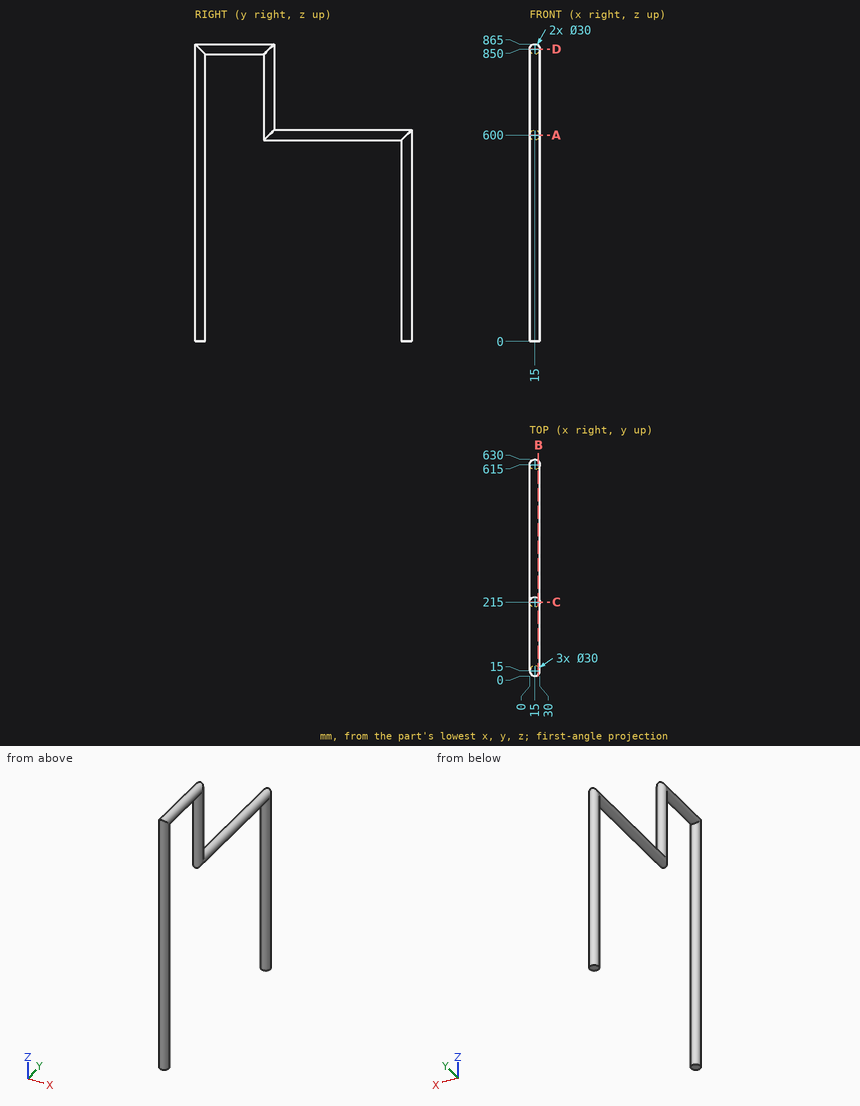
Could you check a few things on this drawing? It's one solid part, dimensions in mm from its lowest x, y, z. Coordinates: 2 decimals unless noted, no trailing zeros. Write each loop counter-clockwise with the first axis right and the second up, starting at its lowest first coordinate (ties: lowest second). Pieces come first, ordered by that corner, then holes. Notation, with made-up numbers: (-1.75, 49.5) - (28.25, 49.5) arc R23 cw to (28.25, 70.5) - close; hole circle Ø6 at (77, 20). An arc over 180 degrees is marked (long way). Return JSON: item names as keys, results as strings. Group by question number.
Item 1: If we section it at D-D (z = 850): Write out the boundary of the cut face in (x, y).
Item 2: I'm going to push flat-ended pins straight in: pin 1 Ø10 at (x, y) = (20, 438.5) entering from +Z; pin 2 Ø10 at (x, z) = (14.5, 307.5) entering from +Y; pin 3 Ø1.5 at (x, z) = (12, 713) entering from -Y; pin 4 Ø6 at (x, z) = (21.5, 559) entering from -Y. Where does each tip first touch, or does it pass through?
Item 3: If we section it at A-A (z = 600): Write out the boundary of the cut face in (x, y), then the cut area to 3 significant figures.
Item 4: Please list where these lines run through material, in increasing order: probe 1 along Y at (x, z) = (13, 750.5); probe 2 along Y at (x, z) = (14, 261); probe 3 along Z at (x, y) = (13.5, 574).
Item 5: If we section it at B-B (x = 25.25): Write out the boundary of the cut face in (y, z).
Item 6: If we section it at C-C (y = 215): Write out the boundary of the cut face in (x, z), then the cut area to 3 significant figures.
Return value:
{
 "1": {"outline": "(0, 15) arc R15 ccw to (30, 15) - (30, 215) arc R15 ccw to (0, 215) - close"},
 "2": {"pin 1": "stops at z = 615", "pin 2": "stops at y = 630", "pin 3": "stops at y = 0.17", "pin 4": "stops at y = 0.41"},
 "3": {"outline": "circle Ø30 at (15, 15); (0, 215) arc R15 ccw to (30, 215) - (30, 615) arc R15 ccw to (0, 615) - close", "area": "13,400 mm^2"},
 "4": {"probe 1": "y = 0.13 to 29.87, 200.13 to 229.87", "probe 2": "y = 0.03 to 29.97, 600.03 to 629.97", "probe 3": "z = 585.08 to 614.92"},
 "5": {"outline": "(4.05, 0) - (25.95, 0) - (25.95, 839.05) - (204.05, 839.05) - (204.05, 589.05) - (604.05, 589.05) - (604.05, 0) - (625.95, 0) - (625.95, 610.95) - (225.95, 610.95) - (225.95, 860.95) - (4.05, 860.95) - close"},
 "6": {"outline": "(0, 600) arc R15 ccw to (30, 600) - (30, 850) arc R15 ccw to (0, 850) - close", "area": "8,210 mm^2"}
}
